Could you check a few things on this drawing? It's one solid part, dimensions in mm from its lowest x, y, z. Give positions to 0.01 mm unless a question says otherwise; leave off trailing zeros. Write each loop counter-clockwise with the first axis right and the second up, starting at its lowest first coordinate (ties: lowest second). Pieces come first, ordered by that corner, then holes. Notation, with made-up numbers: (62, -10.75) - (75, -10.75) arc R19 ccw to (75, 9.25) - close; hole circle Ø10 at (39.5, 47.25). An arc over 180 degrees is marked (long way). One line per item, written item: value. Start each with the question number.
1) I'm going to push flat-ended pins straight in: P1, Ø3.5, axis at y = 10.5, z = 1.5, coming from the +X side; P2, Ø4, axis at x = 6.5, y = 10, coming from the -Z side; P3, Ø5, axis at y = 14.5, z = 20, coming from the +X side; P4, Ø2.5, axis at x = 4.5, z = 18.5, coming from the -Y side. Where does each tip first touch, or does it pass through?
2) Please list where these lines run through material, in increasing order: L1, parallel to Z at x = 5.5, y = 2.75; L2, parallel to X at y = 10.5, z = 28; L3, parallel to Y at x = 7, z = 13. Write a range as [from, to].
3) Imagine slicing it at C-C on z = 25. Write out the boundary of the cut face in (x, y), plus the area to 3 significant figures.
4) We'd pull the mould along Z, two halves only. Please class the marked faces 1, 2, 3 and 4: +Z half, -Z half, draft (parallel to the pull), parting line (faces both ways), or undercut.
5) Imagine slicing it at A-A on x = 7. Write out the boundary of the cut face in (y, z).
6) Imagine slicing it at D-D on x = 3.5. Write out the boundary of the cut face in (y, z), plus the area to 3 significant figures.
7) Imagine slicing it at B-B on y = 2. Write out the boundary of the cut face in (x, z), plus the area to 3 significant figures.
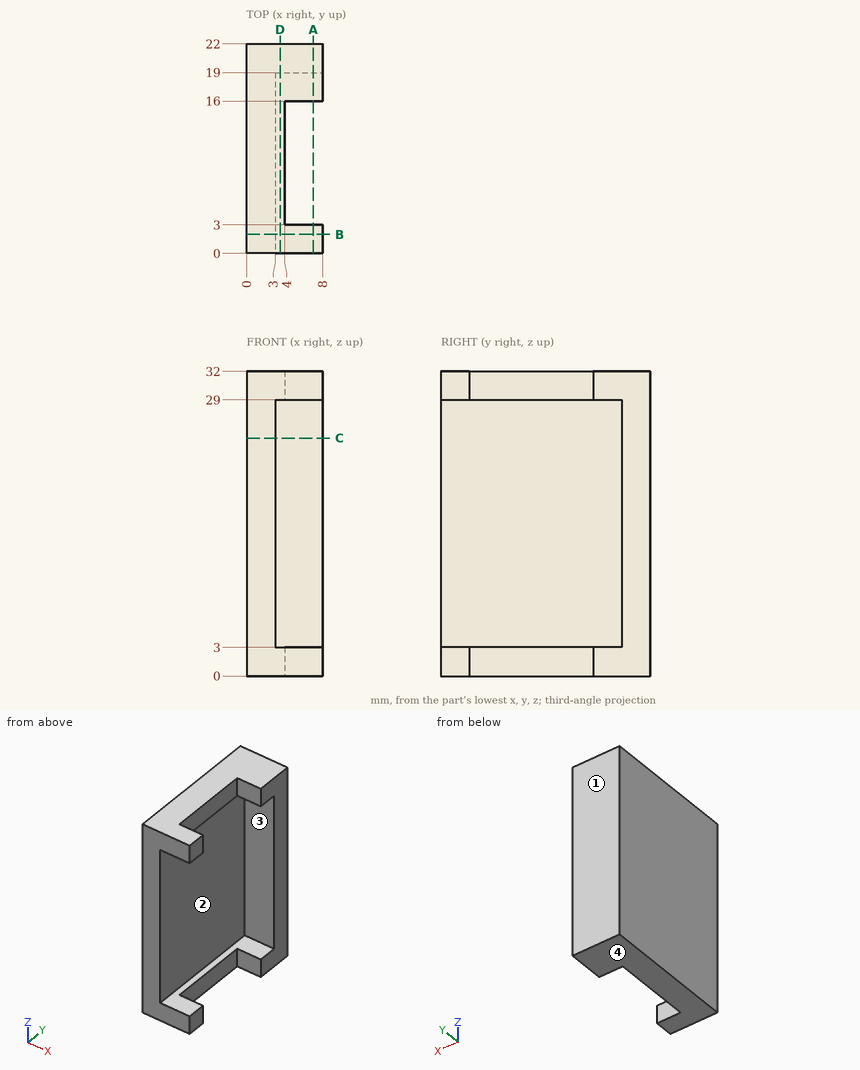
Numbers:
1. P1: x = 4
1. P2: through
1. P3: x = 3
1. P4: y = 19
2. L1: [0, 3], [29, 32]
2. L2: [0, 3]
2. L3: [19, 22]
3. outline: (0, 0) - (3, 0) - (3, 19) - (8, 19) - (8, 22) - (0, 22) - close
3. area: 81.0 mm^2
4. face 1: draft
4. face 2: undercut
4. face 3: undercut
4. face 4: -Z half
5. outline: (0, 0) - (3, 0) - (3, 3) - (0, 3) - close; (0, 29) - (3, 29) - (3, 32) - (0, 32) - close; (16, 0) - (22, 0) - (22, 32) - (16, 32) - (16, 29) - (19, 29) - (19, 3) - (16, 3) - close
6. outline: (0, 0) - (22, 0) - (22, 32) - (0, 32) - (0, 29) - (19, 29) - (19, 3) - (0, 3) - close
6. area: 210 mm^2
7. outline: (0, 0) - (8, 0) - (8, 3) - (3, 3) - (3, 29) - (8, 29) - (8, 32) - (0, 32) - close
7. area: 126 mm^2
